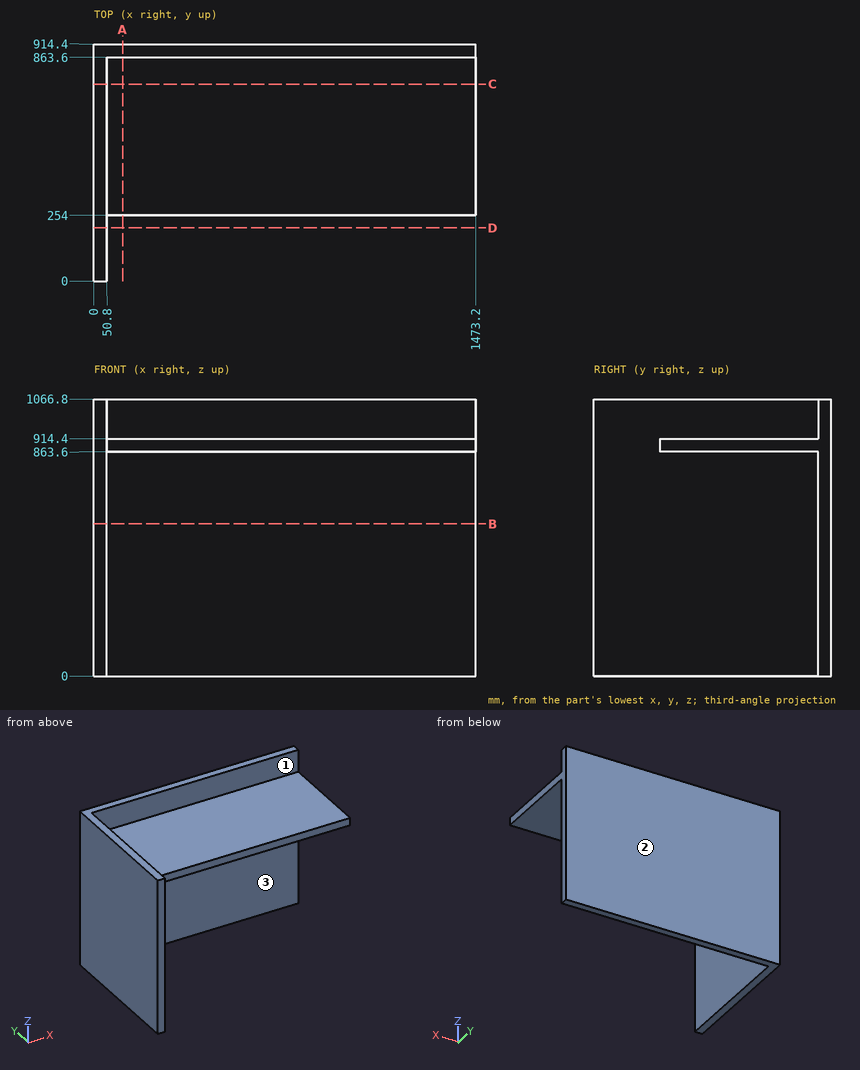
Input: dimensioned drawing with shaded views. Units: mm. Origin: part minimum x, y, z. A direction names the side the tool comes from. Coordinates: 2 decimals unless noted, no trailing zeros. Order: outer loops, then holes, each group sorted by start corner. A loop starts at its lowest first (then second) coordinate and runs counter-clockwise, first axis right, second up. Notation, with made-up numbers: (1, 62) - (19, 62) arc R33 cw to (19, 92) - close; hole circle Ø3 at (1, 12). An arc over 180 degrees is marked (long way). Return JSON: item names as keys, results as strings. Group by question number.
1. Set-up query: the marked faces 1, 2 and 3. Return all of +Z, -Z, +X, -X, +Y, -Y with unobstructed straight access to the full face (end or side cutting, diameter ignored); none if empty.
2. Pin query (flat end, axial travel): pin 1 (1.5 mm diameter, centred on x = 750.5, y = 591.5, fed in from -Z); pin 2 (2 mm diameter, centred on x = 160, y = 425, fed in from +Z); pin 3 (15 mm diameter, centred on x = 842, z = 901, fed in from -Y). Return the tip coordinate at first contact, or that it passes through.
3. Cut plane B-B (z = 586). Output: boundary loops of the cut face in (x, y).
4. Material intervals for line 1 along Y through (x, z) = (600, 981.5); line 2 along X through (y, z) = (43, 846.5), sorted ascending. Write a range as [from, to].
5. Cut plane A-A (x = 111). Output: boundary loops of the cut face in (y, z), plus the area to 3 significant figures.
6. Cut plane D-D (y = 205.5). Output: boundary loops of the cut face in (x, z).
7. Cut plane C-C (y = 760). Output: boundary loops of the cut face in (x, z), plus the area to 3 significant figures.
Resolved:
{
 "1": {"face 1": "+Z, +X, -Y", "face 2": "+Z, -Z, +X, -X, +Y", "face 3": "-Z, +X, -Y"},
 "2": {"pin 1": "stops at z = 863.6", "pin 2": "stops at z = 914.4", "pin 3": "stops at y = 254"},
 "3": {"outline": "(0, 0) - (50.8, 0) - (50.8, 863.6) - (1473.2, 863.6) - (1473.2, 914.4) - (0, 914.4) - close"},
 "4": {"line 1": "y = [863.6, 914.4]", "line 2": "x = [0, 50.8]"},
 "5": {"outline": "(254, 863.6) - (863.6, 863.6) - (863.6, 0) - (914.4, 0) - (914.4, 1066.8) - (863.6, 1066.8) - (863.6, 914.4) - (254, 914.4) - close", "area": "85,200 mm²"},
 "6": {"outline": "(0, 0) - (50.8, 0) - (50.8, 1066.8) - (0, 1066.8) - close"},
 "7": {"outline": "(0, 0) - (50.8, 0) - (50.8, 863.6) - (1473.2, 863.6) - (1473.2, 914.4) - (50.8, 914.4) - (50.8, 1066.8) - (0, 1066.8) - close", "area": "126,000 mm²"}
}
